Read the model definition and answer for the solid it produces. Units are mm, in the model's axes. Face numbers are marked on the shaded views. A direction names the side the tool comes from. Round coordinates to 2 decimals unless told otherwise and drop trailing zeros. Write each loop counter-clockwise with the first axis right and the second up, starting at its lowest first coordinate (ties: lowest second). Pieces come first, ordered by that corner, then holes. Notation, with made-up numbers: (62.5, 9) - (79.5, 9) arc R20 cw to (79.5, 20) - close; hole circle Ø2 at (2.25, -12). An arc over 180 degrees is marked (long way). One line per item, written item: value. Start each with the question number.
(1) Flat-ended cylindrical pins translate along their axes: pin 1 Ø5 at (x, y) = (6, 11) entering from +Z; pin 2 Ø3 at (y, z) = (25, -36) entering from -X; pin 3 Ø9.5 at (y, z) = (30.5, 5) entering from +X. Find the tip coordinate at first contact, or state that the pin passes through.
(2) For the marked faces 1 and 2, determine the directions among +Z, -Z, +X, -X, +Y, -Y from which every point of the face is accessible in a straight line to the end or side of a thin tool.
(3) A cutting plane is placed at D-D, the plane x = 4.75. Determine the outline of the cut face in (y, z).
(4) The mould has two halves that part along Z. Classify the marked faces 3, 4 and 5: +Z half, -Z half, draft (parallel to the pull), parting line (faces both ways), or undercut.
(5) A cutting plane is placed at C-C, the plane y = 3.7. Determine the outline of the cut face in (x, z), plus the area to 3 significant figures.
(6) A cutting plane is placed at B-B, the plane z = -18.5. Determine the outline of the cut face in (x, y), plus the area to 3 significant figures.
(7) Find the intervals of material crossed by L1, parallel to Y at x = 9.75, z = -46.85; L2, parallel to Z at x = 10, y = 41.5; L3, parallel to X at y = 42, z = -8, in increasing order.
(8) A cutting plane is placed at A-A, the plane x = 9.75. Determine the outline of the cut face in (y, z), plus the area to 3 significant figures.
from build123d import *

# Parameters (mm, degrees)
BOSS_EXTRUDE1_DEPTH   = 50
SKETCH3_R             = 1.6
CUT_EXTRUDE1_DEPTH    = 49
SKETCH4_W             = 23.4
SKETCH4_H             = 33
CUT_EXTRUDE2_DEPTH    = 4
FILLET1_R             = 3
FILLET2_R             = 3
F_6_CLEARANCE_HOLE1_D = 3.7973


with BuildPart() as part:
    # Sketch1 → Boss-Extrude1 (new body)
    with BuildSketch(Plane(origin=(0, 0, 0), x_dir=(1, 0, 0), z_dir=(0, 1, 0))):
        Polygon((0, 0), (0, 48), (3, 48), (13, 48), (13, 45), (3, 45), (3, 3), (13, 3), (13, 0), (3, 0), (3, -12), (0, -12), align=None)
    extrude(amount=BOSS_EXTRUDE1_DEPTH)

    # Sketch3 → Cut-Extrude1 (cut, through all)
    with BuildSketch(Plane.XY):
        with Locations((9.75, 43.7)):
            Circle(SKETCH3_R)
        with Locations((9.75, 3.7)):
            Circle(SKETCH3_R)
    extrude(amount=-CUT_EXTRUDE1_DEPTH, mode=Mode.SUBTRACT)

    # Sketch4 → Cut-Extrude2 (cut, through all)
    with BuildSketch(Plane(origin=(3, 0, 0), x_dir=(0, 0, -1), z_dir=(1, 0, 0))):
        with BuildLine():
            Line((0, 50), (-12, 50))
            Line((-12, 50), (-12, 30))
            Line((-12, 30), (-2.878524803, 37.601229331))
            ThreePointArc((-2.878524803, 37.601229331), (-0.75528463, 40.353756398), (0, 43.746999568))
            Line((0, 43.746999568), (0, 50))
        make_face()
        with BuildLine():
            Line((0, 0), (0, 6.253000432))
            ThreePointArc((0, 6.253000432), (-0.75528463, 9.646243602), (-2.878524803, 12.398770669))
            Line((-2.878524803, 12.398770669), (-12, 20))
            Line((-12, 20), (-12, 0))
            Line((-12, 0), (0, 0))
        make_face()
        with Locations((16.3, 22.5)):
            Rectangle(SKETCH4_W, SKETCH4_H)
    extrude(amount=-CUT_EXTRUDE2_DEPTH, mode=Mode.SUBTRACT)

    # Fillet1
    fillet1_edges = [part.edges().sort_by_distance(p)[0] for p in [
        (1.5, 20, 12),
        (1.5, 30, 12),
    ]]
    fillet(fillet1_edges, radius=FILLET1_R)

    # Fillet2
    fillet2_edges = [part.edges().sort_by_distance(p)[0] for p in [
        (1.5, 6, -28),
        (1.5, 6, -4.6),
        (1.5, 39, -4.6),
        (1.5, 39, -28),
    ]]
    fillet(fillet2_edges, radius=FILLET2_R)

    # #6 Clearance Hole1 (through all)
    with Locations(Plane(origin=(3, 0, 0), x_dir=(0, 0, -1), z_dir=(1, 0, 0))):
        with Locations((-6.5, 25), (36, 25)):
            Hole(F_6_CLEARANCE_HOLE1_D / 2)


solid = part.part
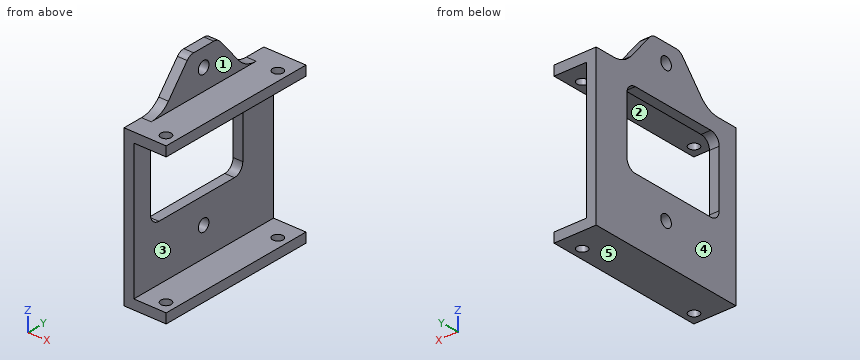
Here are the results:
1. pin 1: z = 0
1. pin 2: through
1. pin 3: x = 3
2. face 1: +Z, +X, +Y, -Y
2. face 2: +X, +Y, -Y
3. outline: (0, -48) - (50, -48) - (50, -45) - (0, -45) - close; (0, -3) - (50, -3) - (50, 0) - (0, 0) - close
4. face 3: undercut
4. face 4: draft
4. face 5: -Z half
5. outline: (0, -48) - (8.15, -48) - (8.15, -45) - (3, -45) - (3, -3) - (8.15, -3) - (8.15, 0) - (0, 0) - close; (11.35, -48) - (13, -48) - (13, -45) - (11.35, -45) - close; (11.35, -3) - (13, -3) - (13, 0) - (11.35, 0) - close
5. area: 185 mm²
6. outline: (0, 0) - (3, 0) - (3, 6) - (0, 6) - close; (0, 39) - (3, 39) - (3, 50) - (0, 50) - close
6. area: 51.0 mm²
7. L1: 0 to 2.1, 5.3 to 42.1, 45.3 to 50
7. L2: -48 to -45, -3 to 0
7. L3: 0 to 3
8. outline: (0, -48) - (2.1, -48) - (2.1, -45) - (0, -45) - close; (0, -3) - (2.1, -3) - (2.1, 0) - (0, 0) - close; (5.3, -48) - (42.1, -48) - (42.1, -45) - (5.3, -45) - close; (5.3, -3) - (42.1, -3) - (42.1, 0) - (5.3, 0) - close; (45.3, -48) - (50, -48) - (50, -45) - (45.3, -45) - close; (45.3, -3) - (50, -3) - (50, 0) - (45.3, 0) - close
8. area: 262 mm²
